```python
from build123d import *

# Parameters (mm, degrees)
SKETCH002_R      = 6
SKETCH002_R_2    = 2.3
EXTRUDE002_DEPTH = 3
SKETCH001_W      = 246
SKETCH001_H      = 46
SKETCH001_W_2    = 240
SKETCH001_H_2    = 40
EXTRUDE001_DEPTH = 30
SKETCH003_R      = 4
SKETCH003_R_2    = 2.3
EXTRUDE003_DEPTH = 5
SKETCH_W         = 246
SKETCH_H         = 46
SKETCH_R         = 3.5
SKETCH_R_2       = 6.1
EXTRUDE_DEPTH    = 3


with BuildPart() as extrude002:
    # Sketch002 (on Face3 of Extrude001) → Extrude002 (new body)
    with BuildSketch(Plane.XZ):
        with Locations((123, 21)):
            Circle(SKETCH002_R)
        with Locations((93.79, 28.16)):
            Circle(SKETCH002_R_2)
        with Locations((93.79, 5.3)):
            Circle(SKETCH002_R_2)
        with Locations((152.21, 5.3)):
            Circle(SKETCH002_R_2)
        with Locations((152.21, 28.16)):
            Circle(SKETCH002_R_2)
    extrude(amount=-EXTRUDE002_DEPTH)


with BuildPart() as cut:
    # Sketch001 (on Face21 of Extrude) → Extrude001 (new body)
    with BuildSketch(Plane.XY.offset(3)):
        with Locations((123, 23)):
            Rectangle(SKETCH001_W, SKETCH001_H)
        with Locations((123, 23)):
            Rectangle(SKETCH001_W_2, SKETCH001_H_2, mode=Mode.SUBTRACT)
    extrude(amount=EXTRUDE001_DEPTH)

    # Cut: cut Extrude002
    add(extrude002.part, mode=Mode.SUBTRACT)


with BuildPart() as extrude003:
    # Sketch003 (on Face6 of Cut) → Extrude003 (new body)
    with BuildSketch(Plane.XZ):
        with Locations((93.79, 28.16)):
            Circle(SKETCH003_R)
        with Locations((93.79, 28.16)):
            Circle(SKETCH003_R_2, mode=Mode.SUBTRACT)
        with Locations((152.21, 28.16)):
            Circle(SKETCH003_R)
        with Locations((152.21, 28.16)):
            Circle(SKETCH003_R_2, mode=Mode.SUBTRACT)
        with Locations((152.21, 5.3)):
            Circle(SKETCH003_R)
        with Locations((152.21, 5.3)):
            Circle(SKETCH003_R_2, mode=Mode.SUBTRACT)
        with Locations((93.79, 5.3)):
            Circle(SKETCH003_R)
        with Locations((93.79, 5.3)):
            Circle(SKETCH003_R_2, mode=Mode.SUBTRACT)
    extrude(amount=EXTRUDE003_DEPTH)


with BuildPart() as fusion:
    # Sketch → Extrude (new body)
    with BuildSketch(Plane.XY):
        with Locations((123, 23)):
            Rectangle(SKETCH_W, SKETCH_H)
        with Locations((12, 23)):
            Circle(SKETCH_R, mode=Mode.SUBTRACT)
        with Locations((24, 23)):
            Circle(SKETCH_R, mode=Mode.SUBTRACT)
        with Locations((36, 23)):
            Circle(SKETCH_R, mode=Mode.SUBTRACT)
        with Locations((54, 23)):
            Circle(SKETCH_R_2, mode=Mode.SUBTRACT)
        with Locations((72, 23)):
            Circle(SKETCH_R_2, mode=Mode.SUBTRACT)
        with Locations((90, 23)):
            Circle(SKETCH_R_2, mode=Mode.SUBTRACT)
        with Locations((108, 23)):
            Circle(SKETCH_R_2, mode=Mode.SUBTRACT)
        with Locations((126, 23)):
            Circle(SKETCH_R_2, mode=Mode.SUBTRACT)
        with Locations((144, 23)):
            Circle(SKETCH_R_2, mode=Mode.SUBTRACT)
        with Locations((162, 23)):
            Circle(SKETCH_R_2, mode=Mode.SUBTRACT)
        with Locations((180, 23)):
            Circle(SKETCH_R_2, mode=Mode.SUBTRACT)
        with Locations((198, 23)):
            Circle(SKETCH_R, mode=Mode.SUBTRACT)
        with Locations((210, 23)):
            Circle(SKETCH_R, mode=Mode.SUBTRACT)
        with Locations((222, 23)):
            Circle(SKETCH_R, mode=Mode.SUBTRACT)
        with Locations((234, 23)):
            Circle(SKETCH_R, mode=Mode.SUBTRACT)
    extrude(amount=EXTRUDE_DEPTH)

    # Fusion: union Cut, Extrude003
    add(cut.part)
    add(extrude003.part)


solid = fusion.part
```
Can you work these out from the model? Positions are in its coordinate system, mm. A direction names the side the tool comes from. Coordinates: 2 decimals unless noted, no trailing zeros. Order: outer loops, then holes, each group sorted by start corner. A loop starts at its lowest first (then second) coordinate and runs counter-clockwise, first axis right, second up. Notation, with made-up numbers: (40.5, -12) - (44.5, -12) arc R24 cw to (44.5, 1) - close; hole circle Ø6 at (-14.75, 72.5). An arc over 180 degrees is marked (long way). Answer in a Markdown table with one row per item.
1. Suppose I cut it at A-A (x = 36). Please give me the cut outline in (y, z), and give its area (3 significant figures).
Reply:
| item | result |
|---|---|
| outline | (0, 0) - (19.5, 0) - (19.5, 3) - (3, 3) - (3, 33) - (0, 33) - close; (26.5, 0) - (46, 0) - (46, 33) - (43, 33) - (43, 3) - (26.5, 3) - close |
| area | 297 mm^2 |
2. For pin 1 (10 mm diameter, centred on x = 180, y = 23, fed in from +Z); pin 2 (2 mm diameter, centred on x = 196.5, z = 28, fed in from -Y); pin 3 (15 mm diameter, centred on y = 29.5, z = 22, fed in from -X); pin 4 (6 mm diameter, centred on x = 116.5, y = 36, fed in from +Z), each with a flat end and sliding along its axis, tell me the tip position at first contact or that it passes through.
Reply:
| item | result |
|---|---|
| pin 1 | passes through |
| pin 2 | stops at y = 0 |
| pin 3 | stops at x = 0 |
| pin 4 | stops at z = 3 |
3. If we mould it in two halves opening along X, with no side actions, what happens to faces 4 (the flat face through (246, 23, 16)), 5 (the cylindrical face through (93.279, 28.144, 1.479)), 6 (the flat face through (96, -5, 26))? For each: pulls with the +X half, pulls with the -X half, needs draft (parallel to the pull), parting line crosses it, or undercut.
Reply:
| item | result |
|---|---|
| face 4 | pulls with the +X half |
| face 5 | undercut |
| face 6 | needs draft |
4. Suppose I cut it at D-D (x = 144). Please give me the cut outline in (y, z), and give its area (3 significant figures).
Reply:
| item | result |
|---|---|
| outline | (0, 0) - (16.9, 0) - (16.9, 3) - (3, 3) - (3, 33) - (0, 33) - close; (29.1, 0) - (46, 0) - (46, 33) - (43, 33) - (43, 3) - (29.1, 3) - close |
| area | 281 mm^2 |
5. For faces 1 (the cylindrical face through (117, 1, 21)), 2 (the cylindrical face through (173.906, 23.268, 1.479)), 3 (the flat face through (121, 3, 14)), which set-ups out of +Z, -Z, +X, -X, +Y, -Y let a thin tool reach every point of the face, with its end or its side?
Reply:
| item | result |
|---|---|
| face 1 | -Y |
| face 2 | +Z, -Z |
| face 3 | +Z |
6. Suppose I cut it at B-B (y = 7). Please give me the cut outline in (x, z).
Reply:
| item | result |
|---|---|
| outline | (0, 0) - (246, 0) - (246, 33) - (243, 33) - (243, 3) - (3, 3) - (3, 33) - (0, 33) - close |
7. If I drill on line 1 along Z through (x, y) = (152.21, -1.4); line 2 along X through (y, z) = (1, 28); line 3 along Y through (x, z) = (182, 19.5), over which ranges is the centre line in solid material (lowest first)?
Reply:
| item | result |
|---|---|
| line 1 | z = 1.3 to 3, 7.6 to 9.3, 24.16 to 25.86, 30.46 to 32.16 |
| line 2 | x = 0 to 91.5, 96.08 to 149.92, 154.5 to 246 |
| line 3 | y = 0 to 3, 43 to 46 |
8. Suppose I cut it at C-C (z = 21). Please give me the cut outline in (x, y), and give its area (3 significant figures).
Reply:
| item | result |
|---|---|
| outline | (0, 0) - (117, 0) - (117, 3) - (3, 3) - (3, 43) - (243, 43) - (243, 3) - (129, 3) - (129, 0) - (246, 0) - (246, 46) - (0, 46) - close |
| area | 1,680 mm^2 |
